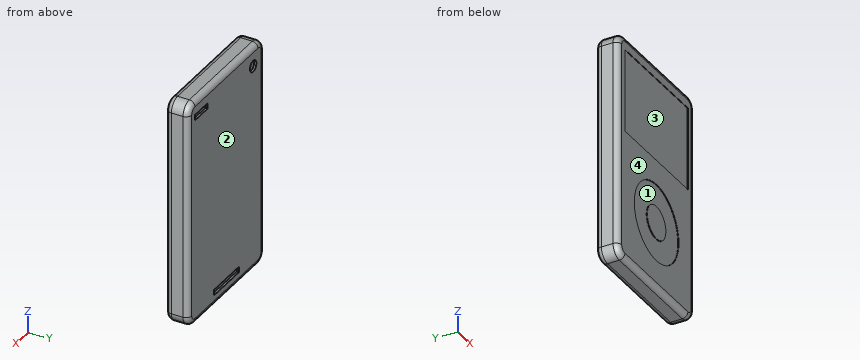
```python
from build123d import *

# Parameters (mm, degrees)
F0_R     = 17.78
F0_W     = 50.8
F0_H     = 38.1
F0_R_2   = 7.62
F1_DEPTH = 10.414
F2_DEPTH = 0.1
F3_W     = 10.16
F3_H     = 2.54
F3_R     = 2.54
F3_W_2   = 20.32
F4_DEPTH = 1
F5_R     = 2.54


with BuildPart() as f1:
    # F0 (on Front) → F1 (new body)
    with BuildSketch(Plane.XZ):
        with BuildLine():
            ThreePointArc((30.48, 46.99), (28.9921024484, 50.5821024484), (25.4, 52.07))
            Line((25.4, 52.07), (-25.4, 52.07))
            ThreePointArc((-25.4, 52.07), (-28.9921024484, 50.5821024484), (-30.48, 46.99))
            Line((-30.48, 46.99), (-30.48, -46.99))
            ThreePointArc((-30.48, -46.99), (-28.9921024484, -50.5821024484), (-25.4, -52.07))
            Line((-25.4, -52.07), (25.4, -52.07))
            ThreePointArc((25.4, -52.07), (28.9921024484, -50.5821024484), (30.48, -46.99))
            Line((30.48, -46.99), (30.48, 46.99))
        make_face()
        with Locations((0, -21.59)):
            Circle(F0_R, mode=Mode.SUBTRACT)
        with Locations((0, 26.67)):
            Rectangle(F0_W, F0_H, mode=Mode.SUBTRACT)
        with Locations((0, 26.67)):
            Rectangle(F0_W, F0_H)
        with Locations((0, -21.59)):
            Circle(F0_R)
        with Locations((0, -21.59)):
            Circle(F0_R_2, mode=Mode.SUBTRACT)
        with Locations((0, -21.59)):
            Circle(F0_R_2)
    extrude(amount=-F1_DEPTH)

    # F0 (on Front) → F2 (cut)
    with BuildSketch(Plane.XZ):
        with Locations((0, 26.67)):
            Rectangle(F0_W, F0_H)
        with Locations((0, -21.59)):
            Circle(F0_R)
        with Locations((0, -21.59)):
            Circle(F0_R_2, mode=Mode.SUBTRACT)
    extrude(amount=-F2_DEPTH, mode=Mode.SUBTRACT)

    # F3 (on face) → F4 (cut)
    with BuildSketch(Plane(origin=(0, 10.414, 0), x_dir=(-1, 0, 0), z_dir=(0, 1, 0))):
        with Locations((-20.32, 44.45)):
            Rectangle(F3_W, F3_H)
        with Locations((21.59, 43.18)):
            Circle(F3_R)
        with Locations((0, -45.72)):
            Rectangle(F3_W_2, F3_H)
    extrude(amount=-F4_DEPTH, mode=Mode.SUBTRACT)

    # F5
    f5_edges = [f1.edges().sort_by_distance(p)[0] for p in [
        (30.48, 0, 0),
        (30.48, 10.414, 0),
    ]]
    fillet(f5_edges, radius=F5_R)


solid = f1.part
```
The listing builds one solid part. Answer for the finished solid, in the listing's coordinates (mm). Face numbers are marked on the shaded views. A direction names the side the tool comes from. Coordinates: 2 decimals unless noted, no trailing zeros. Loops run counter-clockwise (first coordinate to the right, second up) from the corner with the lowest first, then second, coordinate; pieces in that order, holes last. Notation, with made-up numbers: (-29, 76.5) - (-7, 76.5) arc R14 cw to (-7, 95.5) - close; hole circle Ø3 at (-21.75, -34.5). An arc over 180 degrees is marked (long way). Write item = value, one per line.
1) Each of these flat-tipped pins is pushed along its axis until it touches: P1, Ø6, axis at x = -17.5, z = 32.5, coming from the -Y side; P2, Ø0.5, axis at y = 10, z = -45.5, coming from the -X side; P3, Ø0.8, axis at y = 10, z = 44.5, coming from the +X side; P4, Ø5, axis at x = 11, y = 8, coming from the -Z side. Where does it stop, or does it pass through?
Responses:
P1 = 0.1
P2 = -29.65
P3 = 29.8
P4 = -52.07
2) Determine the mould class of the marked faces 3 and 4 for opening direction Z: pulls with the +Z half, pulls with the -Z half, needs draft (parallel to the pull), parting line crosses it, or undercut.
Responses:
face_3 = undercut
face_4 = needs draft
3) Section B-B (y = 1.25) is taken. Determine the outline of the cut face in (x, z).
Responses:
outline = (-30.13, -46.99) arc R4.73 ccw to (-25.4, -51.72) - (25.4, -51.72) arc R4.73 ccw to (30.13, -46.99) - (30.13, 46.99) arc R4.73 ccw to (25.4, 51.72) - (-25.4, 51.72) arc R4.73 ccw to (-30.13, 46.99) - close
4) Which of the six approach directions +Z, -Z, +X, -X, +Y, -Y give full straight-line access (tool end or side, diameter ignored) to the marked faces 1 and 2?
Responses:
face_1 = -Y
face_2 = +Z, -Z, +X, -X, +Y
5) Find the intervals of material crossed by line 1 along Y through (x, z) = (23, 32); line 2 along Z through (x, y) = (25.5, 8); line 3 along Z through (x, y) = (-21.59, 9.8), in increasing order.
Responses:
line_1 = 0.1 to 10.41
line_2 = -52.07 to 52.07
line_3 = -51.19 to 40.64, 45.72 to 51.19
6) Section A-A (z = 24) is taken. Determine the outline of the cut face in (x, y).
Responses:
outline = (-30.48, 2.54) arc R2.54 ccw to (-27.94, 0) - (-25.4, 0) - (-25.4, 0.1) - (25.4, 0.1) - (25.4, 0) - (27.94, 0) arc R2.54 ccw to (30.48, 2.54) - (30.48, 7.87) arc R2.54 ccw to (27.94, 10.41) - (-27.94, 10.41) arc R2.54 ccw to (-30.48, 7.87) - close
